Job drawing, mm, ordinate dimensions from the low corner. One solid piece. A direction names the side the tool comes from. Give positions to 0.01 mm unless a question says otherwise; leave off trailing zeros. Order: outer loops, then holes, each group sorted by start corner. A loop starts at its lowest first (then second) coordinate and runs counter-clockwise, first axis right, second up. Notation, with made-up numbers: M 84.5,81.5 L 117.5,81.5 A22 cw 117.5,104.5 Z; hole C -23,-20 d4. An arc over 180 degrees is marked long. One line per question, with ' | ' between items.
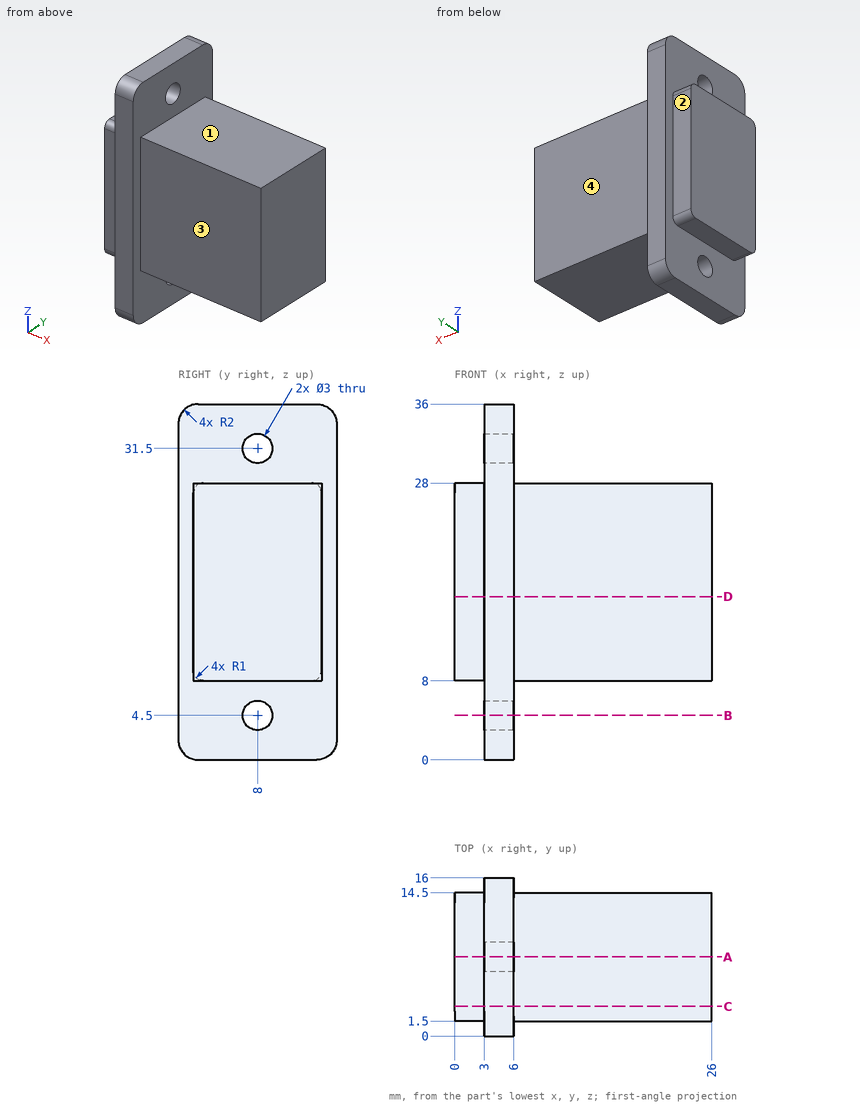
1. Slice it at A-A on y = 8. Give the cut face in (x, z).
Worked out:
outline: M 0,8 L 3,8 L 3,6 L 6,6 L 6,8 L 26,8 L 26,28 L 6,28 L 6,30 L 3,30 L 3,28 L 0,28 Z; M 3,0 L 6,0 L 6,3 L 3,3 Z; M 3,33 L 6,33 L 6,36 L 3,36 Z
2. Drop flat-ended pins along their axis: pin 1 (1.5 mm diameter, centred on x = 21.5, z = 21, fed in from +Y); pin 2 (1.5 mm diameter, centred on x = 1.5, z = 13.5, fed in from -Y); pin 3 (1.5 mm diameter, centred on x = 2, y = 5.5, fed in from +Z); pin 4 (2.5 mm diameter, centred on y = 8, z = 4.5, fed in from -X). Give the stop position or say it passes through.
Worked out:
pin 1: stops at y = 14.5 | pin 2: stops at y = 1.5 | pin 3: stops at z = 28 | pin 4: passes through
3. Slice it at B-B on z = 4.5. Give the cut face in (x, y), then the cut area to 3 significant figures.
Worked out:
outline: M 3,0 L 6,0 L 6,6.5 L 3,6.5 Z; M 3,9.5 L 6,9.5 L 6,16 L 3,16 Z | area: 39.0 mm2
4. Slice it at C-C on y = 3. Give the cut face in (x, z).
Worked out:
outline: M 0,8 L 3,8 L 3,0 L 6,0 L 6,8 L 26,8 L 26,28 L 6,28 L 6,36 L 3,36 L 3,28 L 0,28 Z
5. Slice it at D-D on z = 16.5. Give the cut face in (x, y).
Worked out:
outline: M 0,1.5 L 3,1.5 L 3,0 L 6,0 L 6,1.5 L 26,1.5 L 26,14.5 L 6,14.5 L 6,16 L 3,16 L 3,14.5 L 0,14.5 Z
6. Probe L1, parallel to Y at x = 4.55, z = 4.5; L2, parallel to X at y = 14.5, z = 3; L3, parallel to Z at x = 23.75, y = 8.75. List the from-to ranges inside material, lowest first. Write a range as from..to.
Worked out:
L1: y = 0..6.5, 9.5..16 | L2: x = 3..6 | L3: z = 8..28
7. Tool access for the marked faces 1, 2, 3 and 4: list every direction of +Z, -Z, +X, -X, +Y, -Y with a clear straight run to the whole face (end or side of a thin tool).
Worked out:
face 1: +Z, +X, +Y, -Y | face 2: +Z, -Z, -X, +Y | face 3: +Z, -Z, +X, -Y | face 4: +Z, -Z, +X, +Y
